Read the model definition and answer for the solid it produces. Units are mm, in the model's axes. A direction names the side the tool comes from. Round coordinates to 2 decimals unless told otherwise and drop trailing zeros. Write each loop counter-clockwise with the first axis right and the second up, starting at its lowest first coordinate (ties: lowest second). Pieces come first, ordered by that corner, then holes.
from build123d import *

# Parameters (mm, degrees)
BOSS_EXTRUDE7_DEPTH  = 25
SKETCH1_12_W         = 60
SKETCH1_12_H         = 10
BOSS_EXTRUDE8_DEPTH  = 20
BOSS_EXTRUDE9_DEPTH  = 40
BOSS_EXTRUDE10_DEPTH = 20


with BuildPart() as part:
    # Sketch1 → Boss-Extrude7 (new body)
    with BuildSketch(Plane(origin=(0, 0, 0), x_dir=(0, 0, -1), z_dir=(1, 0, 0))):
        Polygon((60, 20), (30, 30), (30, 20), align=None)
    extrude(amount=BOSS_EXTRUDE7_DEPTH)



with BuildPart() as body_2:
    # Sketch1_12 → Boss-Extrude8 (new body)
    with BuildSketch(Plane(origin=(0, 0, 0), x_dir=(0, 0, -1), z_dir=(1, 0, 0))):
        with Locations((30, -5)):
            Rectangle(SKETCH1_12_W, SKETCH1_12_H)
    extrude(amount=BOSS_EXTRUDE8_DEPTH)


with BuildPart() as part_1:
    add(part.part)

    add(body_2.part)  # Boss-Extrude9 merges body 2
    # Sketch1_13 → Boss-Extrude9 (add)
    with BuildSketch(Plane(origin=(0, 0, 0), x_dir=(0, 0, -1), z_dir=(1, 0, 0))):
        Polygon((30, 30), (0, 40), (0, 0), (60, 0), (60, 20), (30, 20), align=None)
    extrude(amount=BOSS_EXTRUDE9_DEPTH)

    # Sketch1_14 → Boss-Extrude10 (add)
    with BuildSketch(Plane(origin=(0, 0, 0), x_dir=(0, 0, -1), z_dir=(1, 0, 0))):
        Polygon((0, 50), (60, 30), (60, 20), (0, 40), align=None)
        Polygon((30, 30), (0, 40), (0, 0), (60, 0), (60, 20), (30, 20), align=None)
        Polygon((60, 20), (30, 30), (30, 20), align=None)
    extrude(amount=-BOSS_EXTRUDE10_DEPTH)


solid = part_1.part
Q1. Which of the six approach directions +Z, -Z, +X, -X, +Y, -Y give full straight-line access (tool end or side, diameter ignored) to faces 1 (the flat face through (40, 16, -23)), 2 (the flat face through (-10, 40, -30)), 3 (the flat face through (32, 20, -45)), 4 (the flat face through (-10, 0, -30)), 5 (the flat face through (30, 0, -30))?
Verdict:
face 1: +Z, -Z, +X, +Y, -Y
face 2: -Z, +X, -X, +Y
face 3: -Z, +X, +Y
face 4: +Z, -Z, -X, -Y
face 5: +Z, -Z, +X, -Y
Q2. Straight lines are drawn through the part: probe 1 along X at (y, z) = (-5.5, -43.5); probe 2 along X at (y, z) = (21, -41). For each, find the intervals that lie inside material, in ascending order.
Verdict:
probe 1: x = 0 to 20
probe 2: x = -20 to 25
Q3. Determine the mould class of faces 6 (the flat face through (0, -5, -30)), 7 (the flat face through (10, 10, -60)), 8 (the flat face through (20, -5, -30)) for opening direction X: pulls with the +X half, pulls with the -X half, needs draft (parallel to the pull), parting line crosses it, or undercut.
Verdict:
face 6: pulls with the -X half
face 7: needs draft
face 8: pulls with the +X half
Q4. Section D-D (z = -22.5) is taken. Determine the outline of the cut face in (x, y).
Verdict:
outline: (-20, 0) - (0, 0) - (0, -10) - (20, -10) - (20, 0) - (40, 0) - (40, 32.5) - (0, 32.5) - (0, 42.5) - (-20, 42.5) - close
Q5. Section B-B (y = 21) is taken. Determine the outline of the cut face in (x, z).
Verdict:
outline: (-20, -60) - (0, -60) - (0, -57) - (25, -57) - (25, -30) - (40, -30) - (40, 0) - (-20, 0) - close
Q6. Section C-C (x = 28.5) is taken. Determine the outline of the cut face in (y, z), then the cut area to 3 significant figures.
Verdict:
outline: (0, -60) - (20, -60) - (20, -30) - (30, -30) - (40, 0) - (0, 0) - close
area: 1,650 mm2
Q7. Flat-ended cylindrical pins translate along their axes: pin 1 Ø10 at (x, z) = (31, -51.5) entering from -Y; pin 2 Ø5 at (y, z) = (23, -45) entering from +X; pin 3 Ø8 at (y, z) = (-7.5, -18.5) entering from +X. Find the tip coordinate at first contact, or state that the pin passes through.
Verdict:
pin 1: stops at y = 0
pin 2: stops at x = 25
pin 3: stops at x = 20
Q8. Section A-A (z = -31.5) is taken. Determine the outline of the cut face in (x, y), then the cut area to 3 significant figures.
Verdict:
outline: (-20, 0) - (0, 0) - (0, -10) - (20, -10) - (20, 0) - (40, 0) - (40, 20) - (25, 20) - (25, 29.5) - (0, 29.5) - (0, 39.5) - (-20, 39.5) - close
area: 2,030 mm2
